```python
from build123d import *

# Parameters (mm, degrees)
SKETCH2_W  = 5.6
SKETCH2_H  = 0.8
SLOT_DEPTH = 0.7


with BuildPart() as part:
    # Fillet2: read off the stored shape, not the designer's step
    # Fillet2 outline → Fillet2 (revolve)
    with BuildSketch(Plane.YX):
        with BuildLine():
            Line((1.5, 1.8), (1.5, 31.8))
            Line((1.5, 31.8), (0, 31.8))
            Line((0, 31.8), (0, 0))
            Line((0, 0), (1.817822349, 0))
            ThreePointArc((1.817822349, 0), (2.425853536, 0.236450397), (2.714397577, 0.821559832))
            Line((2.714397577, 0.821559832), (2.8, 1.8))
            Line((2.8, 1.8), (1.5, 1.8))
        make_face()
    revolve(axis=Axis((0, 0, 0), (1, 0, 0)))

    # Sketch2 → Slot (cut)
    with BuildSketch(Plane(origin=(0, 0, 0), x_dir=(0, 0, -1), z_dir=(1, 0, 0))):
        Rectangle(SKETCH2_W, SKETCH2_H)
    extrude(amount=SLOT_DEPTH, mode=Mode.SUBTRACT)


solid = part.part
```
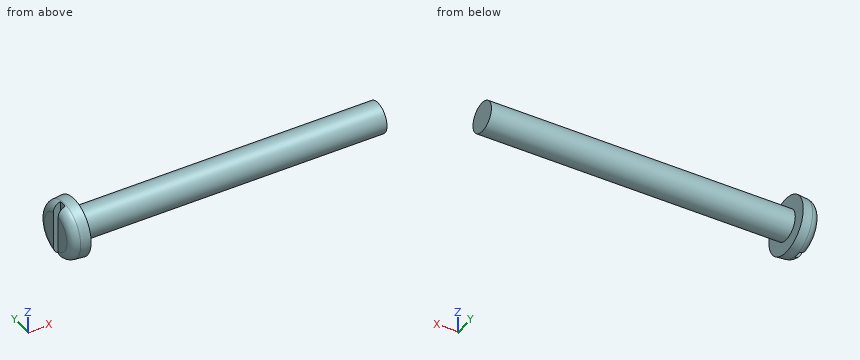
Source: CAD feature listing. Evaluate the final solid. Frame: model axes, mm. Give positions to 0.01 mm unless a question says otherwise; leave off trailing zeros. Loops run counter-clockwise (first coordinate to the right, second up) from the corner with the lowest first, then second, coordinate; pieces in that order, holes last. Notation, with made-up numbers: (65, 15.5) -> (105, 15.5) arc R21 cw to (105, 27.5) -> close; hole circle Ø1 at (87.5, -32). An arc over 180 degrees is marked (long way). Use a Markdown table: item, result. Add a question column.
(1) Section query B-B (y = 0). Output: boundary loops of the cut face in (x, z), then the cut area to 3 significant figures.
(2) Section query C-C (x = 17). Output: boundary loops of the cut face in (y, z), then the cut area to 3 significant figures.
(3) First-contact query: pin 1 Ø2 at (x, y) = (6, -1.5) entering from -Z; pin 2 Ø1.5 at (x, y) = (23.5, 1) entering from +Z. Flat tips, straight axial feed; report the tip coordinate or a pass-through.
(4) Ray query, line 1 (X direction, y = 0.7, z = 1.7); line 2 (Z direction, x = 18.5, y = 1.2); line 3 (Y direction, x = 30, z = 1.1). Return the intervals inside material, ascending.
(5) Section query A-A (z = 0). Output: boundary loops of the cut face in (x, y), then the cut area to 3 significant figures.
Checked values:
| question | item | result |
|---|---|---|
| 1 | outline | (0.7, -2.7) arc R0.9 ccw to (0.82, -2.71) -> (1.8, -2.8) -> (1.8, -1.5) -> (31.8, -1.5) -> (31.8, 1.5) -> (1.8, 1.5) -> (1.8, 2.8) -> (0.82, 2.71) arc R0.9 ccw to (0.7, 2.7) -> close |
| 1 | area | 96.1 mm^2 |
| 2 | outline | circle Ø3 at (0, 0) |
| 2 | area | 7.07 mm^2 |
| 3 | pin 1 | z = -1.41 |
| 3 | pin 2 | z = 1.48 |
| 4 | line 1 | 0 to 1.8 |
| 4 | line 2 | -0.9 to 0.9 |
| 4 | line 3 | -1.02 to 1.02 |
| 5 | outline | (0, -1.82) arc R0.9 ccw to (0.82, -2.71) -> (1.8, -2.8) -> (1.8, -1.5) -> (31.8, -1.5) -> (31.8, 1.5) -> (1.8, 1.5) -> (1.8, 2.8) -> (0.82, 2.71) arc R0.9 ccw to (0, 1.82) -> (0, 0.4) -> (0.7, 0.4) -> (0.7, -0.4) -> (0, -0.4) -> close |
| 5 | area | 99.0 mm^2 |
